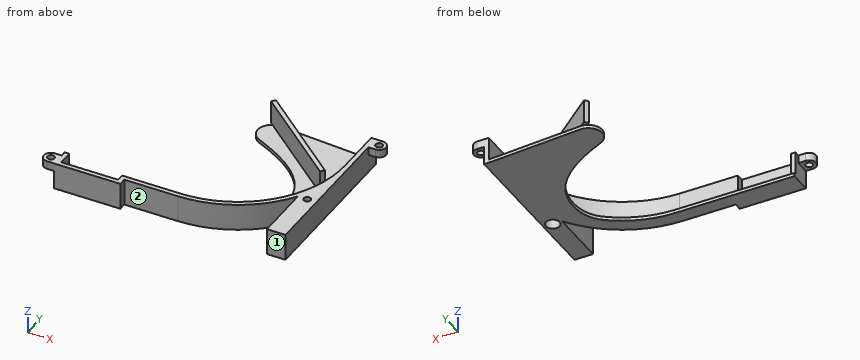
from build123d import *

# Parameters (mm, degrees)
BOSS_EXTRUDE1_DEPTH = 10
BOSS_EXTRUDE2_DEPTH = 1.5
BOSS_EXTRUDE4_DEPTH = 10
SKETCH4_R           = 1.5
BOSS_EXTRUDE3_DEPTH = 11.5
SKETCH5_R           = 1.5
SKETCH5_R_2         = 3
CUT_EXTRUDE1_DEPTH  = 8


with BuildPart() as part:
    # Sketch1 → Boss-Extrude1 (new body)
    with BuildSketch(Plane.XY):
        with BuildLine():
            Line((23.126155741, 11.486298975), (23.126155741, -9.296311409))
            ThreePointArc((23.126155741, -9.296311409), (9.625591469, -41.889556774), (-22.967653896, -55.390121046))
            Line((-22.967653896, -55.390121046), (-48.04069211, -55.390121046))
            Line((-48.04069211, -55.390121046), (-48.04069211, -58.565121046))
            Line((-48.04069211, -58.565121046), (-72.54069211, -58.565121046))
            Line((-72.54069211, -58.565121046), (-72.54069211, -52.215121046))
            Line((-72.54069211, -52.215121046), (-74.54069211, -52.215121046))
            Line((-74.54069211, -52.215121046), (-74.54069211, -60.565121046))
            Line((-74.54069211, -60.565121046), (-46.04069211, -60.565121046))
            Line((-46.04069211, -60.565121046), (-46.04069211, -57.390121046))
            Line((-46.04069211, -57.390121046), (-22.967653896, -57.390121046))
            ThreePointArc((-22.967653896, -57.390121046), (11.039805031, -43.303770336), (25.126155741, -9.296311409))
            Line((25.126155741, -9.296311409), (25.126155741, 11.486298975))
            Line((25.126155741, 11.486298975), (23.126155741, 11.486298975))
        make_face()
    extrude(amount=BOSS_EXTRUDE1_DEPTH)

    # Sketch2 → Boss-Extrude2 (add)
    with BuildSketch(Plane(origin=(0, 0, 0), x_dir=(-1, 0, 0), z_dir=(0, 0, -1))):
        with BuildLine():
            Line((-23.126155741, 11.486298975), (17.693603893, 14.436753165))
            ThreePointArc((17.693603893, 14.436753165), (23.933278885, 9.961444684), (20.661865311, 3.014518513))
            add(Edge.make_bspline(
                [(20.661865311, 3.014518513), (14.467019278, 0.125814366), (-11.141513341, -11.233209967), (-9.492969782, -37.302039453), (-3.109665986, -42.33964958)],
                knots=[0, 0, 0, 0, 0.582936219, 1, 1, 1, 1], degree=3))
            ThreePointArc((-3.109665986, -42.33964958), (9.166044877, -49.06318705), (22.967653896, -51.390121046))
            Line((22.967653896, -51.390121046), (52.04069211, -51.390121046))
            Line((52.04069211, -51.390121046), (74.54069211, -51.390121046))
            Line((74.54069211, -51.390121046), (74.54069211, -52.215121046))
            Line((74.54069211, -52.215121046), (74.54069211, -60.565121046))
            Line((74.54069211, -60.565121046), (46.04069211, -60.565121046))
            Line((46.04069211, -60.565121046), (46.04069211, -57.390121046))
            Line((46.04069211, -57.390121046), (22.967653896, -57.390121046))
            ThreePointArc((22.967653896, -57.390121046), (-11.039805031, -43.303770336), (-25.126155741, -9.296311409))
            Line((-25.126155741, -9.296311409), (-25.126155741, 11.486298975))
            Line((-25.126155741, 11.486298975), (-23.126155741, 11.486298975))
        make_face()
    extrude(amount=BOSS_EXTRUDE2_DEPTH)

    # Sketch6 → Boss-Extrude4 (add)
    with BuildSketch(Plane.XY):
        Polygon((-21.765334092, 14.753493125), (16.605109206, -17.304408883), (17.887425286, -15.769591151), (-20.483018011, 16.288310857), align=None)
    extrude(amount=BOSS_EXTRUDE4_DEPTH)

    # Sketch4 → Boss-Extrude3 (add)
    with BuildSketch(Plane(origin=(0, 0, -1.5), x_dir=(-1, 0, 0), z_dir=(0, 0, -1))):
        with BuildLine():
            Line((-25.126155741, -9.296311409), (-25.126155741, -60.565121046))
            Line((-25.126155741, -60.565121046), (-17.126155741, -60.565121046))
            Line((-17.126155741, -60.565121046), (-17.126155741, -35.857579341))
            ThreePointArc((-17.126155741, -35.857579341), (-23.082745525, -23.166251515), (-25.126155741, -9.296311409))
        make_face()
        with Locations((-21.147916143, -35.857579341)):
            Circle(SKETCH4_R, mode=Mode.SUBTRACT)
        with BuildLine():
            Line((-28.126155741, 11.486298975), (-25.126155741, 11.486298975))
            Line((-25.126155741, 11.486298975), (-25.126155741, 5.486298975))
            Line((-25.126155741, 5.486298975), (-28.126155741, 5.486298975))
            ThreePointArc((-28.126155741, 5.486298975), (-31.126155741, 8.486298975), (-28.126155741, 11.486298975))
        make_face()
        with Locations((-28.126155741, 8.486298975)):
            Circle(SKETCH4_R, mode=Mode.SUBTRACT)
        with BuildLine():
            Line((74.54069211, -60.565121046), (74.54069211, -54.565121046))
            Line((74.54069211, -54.565121046), (77.54069211, -54.565121046))
            ThreePointArc((77.54069211, -54.565121046), (80.54069211, -57.565121046), (77.54069211, -60.565121046))
            Line((77.54069211, -60.565121046), (74.54069211, -60.565121046))
        make_face()
        with Locations((77.54069211, -57.565121046)):
            Circle(SKETCH4_R, mode=Mode.SUBTRACT)
    extrude(amount=-BOSS_EXTRUDE3_DEPTH)

    # Sketch5 → Cut-Extrude1 (cut)
    with BuildSketch(Plane(origin=(0, 0, -1.5), x_dir=(-1, 0, 0), z_dir=(0, 0, -1))):
        with BuildLine():
            Line((77.54069211, -54.565121046), (74.54069211, -54.565121046))
            Line((74.54069211, -54.565121046), (74.54069211, -60.565121046))
            Line((74.54069211, -60.565121046), (77.54069211, -60.565121046))
            ThreePointArc((77.54069211, -60.565121046), (80.54069211, -57.565121046), (77.54069211, -54.565121046))
        make_face()
        with Locations((77.54069211, -57.565121046)):
            Circle(SKETCH5_R, mode=Mode.SUBTRACT)
        with Locations((-21.147916143, -35.857579341)):
            Circle(SKETCH5_R_2)
        with Locations((-21.147916143, -35.857579341)):
            Circle(SKETCH5_R, mode=Mode.SUBTRACT)
        with BuildLine():
            Line((-28.126155741, 5.486298975), (-25.126155741, 5.486298975))
            Line((-25.126155741, 5.486298975), (-25.126155741, 11.486298975))
            Line((-25.126155741, 11.486298975), (-28.126155741, 11.486298975))
            ThreePointArc((-28.126155741, 11.486298975), (-31.126155741, 8.486298975), (-28.126155741, 5.486298975))
        make_face()
        with Locations((-28.126155741, 8.486298975)):
            Circle(SKETCH5_R, mode=Mode.SUBTRACT)
    extrude(amount=-CUT_EXTRUDE1_DEPTH, mode=Mode.SUBTRACT)


solid = part.part
Design review of the part built by this model. Coordinates are the model's own, in mm. Face numbers are marked on the shaded views. Round coordinates to 2 decimals unless told otherwise and drop trailing zeros. Write each loop counter-clockwise with the first axis right and the second up, starting at its lowest first coordinate (ties: lowest second). Pieces come first, ordered by that corner, then holes. Notation, with made-up numbers: (63.25, 33) -> (75.25, 33) arc R10 ccw to (75.25, 49) -> close; hole circle Ø11 at (81.25, 74.25). An arc over 180 degrees is marked (long way). One line per item, written item: value. Start each with the question number.
Q1. The part is to be moulded in two halves that separate along X. For the marked faces 1 and 2, say which applies: pulls with the +X half, pulls with the -X half, needs draft (parallel to the pull), parting line crosses it, or undercut.
Q2. Add section A-A (z = 1.5). Give the boundary of the cut face in (x, y).
Q3. Add section B-B (x = -42.5). Give the boundary of the cut face in (y, z), then the cut area to 3 significant figures.
Q4. Insertion check: P1, Ø0.6, axis at x = -74, z = 3.5, coming from the +Y side; P2, Ø3.5, axis at x = -77.54, y = -57.57, coming from the -Z side; P3, Ø3.5, axis at y = -56.5, z = 5, coming from the -X side. Each pin has a flat end and moves straight along its axis. Give the tip position at first contact, or say it passes through.
Q5. To check wall thickness, follow probe 1 along X at (y, z) = (-37.5, 3); probe 2 along Y at (x, z) = (8, 4.25); probe 3 along Y at (x, z) = (-44, 1). State the ranges of each line that lie inside material, in increasing order.
Response:
1. face 1: needs draft
1. face 2: undercut
2. outline: (-74.54, -60.57) -> (-46.04, -60.57) -> (-46.04, -57.39) -> (-22.97, -57.39) arc R48.09 ccw to (17.13, -35.86) -> (17.13, -60.57) -> (25.13, -60.57) -> (25.13, 11.49) -> (23.13, 11.49) -> (23.13, -9.3) arc R46.09 cw to (-22.97, -55.39) -> (-48.04, -55.39) -> (-48.04, -58.57) -> (-72.54, -58.57) -> (-72.54, -52.22) -> (-74.54, -52.22) -> close; (-21.77, 14.75) -> (16.61, -17.3) -> (17.89, -15.77) -> (-20.48, 16.29) -> close; hole circle Ø6 at (21.15, -35.86)
3. outline: (-57.39, -1.5) -> (-51.39, -1.5) -> (-51.39, 0) -> (-55.39, 0) -> (-55.39, 10) -> (-57.39, 10) -> close
3. area: 29.0 mm^2
4. P1: stops at y = -52.22
4. P2: stops at z = 6.5
4. P3: stops at x = -80.54
5. probe 1: x = 13.49 to 15.99, 17.13 to 18.64, 23.66 to 25.13
5. probe 2: y = -46.09 to -43.44, -10.11 to -7.51
5. probe 3: y = -57.39 to -55.39
